from build123d import *

# Parameters (mm, degrees)
SKETCH1_W           = 54
SKETCH1_H           = 90
SKETCH1_W_2         = 38
SKETCH1_H_2         = 74
BOSS_EXTRUDE1_DEPTH = 40
CUT_EXTRUDE1_DEPTH  = 4.1
CUT_EXTRUDE2_DEPTH  = 0.5
CUT_EXTRUDE3_DEPTH  = 4.1
SKETCH7_R           = 4.1
CUT_EXTRUDE4_DEPTH  = 0.5
SKETCH8_W           = 54
SKETCH8_H           = 90
BOSS_EXTRUDE2_DEPTH = 2
SKETCH9_W           = 54
SKETCH9_H           = 90
BOSS_EXTRUDE3_DEPTH = 2


with BuildPart() as part:
    # Sketch1 → Boss-Extrude1 (new body)
    with BuildSketch(Plane.XY):
        with Locations((27, 45)):
            Rectangle(SKETCH1_W, SKETCH1_H)
        with Locations((27, 45)):
            Rectangle(SKETCH1_W_2, SKETCH1_H_2, mode=Mode.SUBTRACT)
    extrude(amount=BOSS_EXTRUDE1_DEPTH)

    # Sketch2 → Cut-Extrude1 (cut)
    with BuildSketch(Plane.ZY.offset(-46)):
        Polygon((25.888972746, 63), (22.944486373, 68.1), (17.055513627, 68.1), (14.111027254, 63), (17.055513627, 57.9), (22.944486373, 57.9), align=None)
        Polygon((25.888972746, 27), (22.944486373, 32.1), (17.055513627, 32.1), (14.111027254, 27), (17.055513627, 21.9), (22.944486373, 21.9), align=None)
    extrude(amount=-CUT_EXTRUDE1_DEPTH, mode=Mode.SUBTRACT)

    # Sketch5 → Cut-Extrude2 (cut)
    with BuildSketch(Plane.ZY.offset(-50.1)):
        Polygon((17.632863896, 22.9), (22.367136104, 22.9), (24.734272207, 27), (22.367136104, 31.1), (17.632863896, 31.1), (15.265727793, 27), align=None)
        Polygon((24.734272207, 63), (22.367136104, 67.1), (17.632863896, 67.1), (15.265727793, 63), (17.632863896, 58.9), (22.367136104, 58.9), align=None)
    extrude(amount=-CUT_EXTRUDE2_DEPTH, mode=Mode.SUBTRACT)

    # Sketch6 → Cut-Extrude3 (cut)
    with BuildSketch(Plane(origin=(8, 0, 0), x_dir=(0, 0, -1), z_dir=(1, 0, 0))):
        Polygon((-14.111027254, 63), (-17.055513627, 68.1), (-22.944486373, 68.1), (-25.888972746, 63), (-22.944486373, 57.9), (-17.055513627, 57.9), align=None)
        Polygon((-14.111027254, 27), (-17.055513627, 32.1), (-22.944486373, 32.1), (-25.888972746, 27), (-22.944486373, 21.9), (-17.055513627, 21.9), align=None)
    extrude(amount=-CUT_EXTRUDE3_DEPTH, mode=Mode.SUBTRACT)

    # Sketch7 → Cut-Extrude4 (cut)
    with BuildSketch(Plane(origin=(3.9, 0, 0), x_dir=(0, 0, -1), z_dir=(1, 0, 0))):
        with Locations((-20, 63)):
            Circle(SKETCH7_R)
        with Locations((-20, 27)):
            Circle(SKETCH7_R)
    extrude(amount=-CUT_EXTRUDE4_DEPTH, mode=Mode.SUBTRACT)

    # Sketch8 → Boss-Extrude2 (add)
    with BuildSketch(Plane.XY.offset(40)):
        with Locations((27, 45)):
            Rectangle(SKETCH8_W, SKETCH8_H)
    extrude(amount=BOSS_EXTRUDE2_DEPTH)

    # Sketch9 → Boss-Extrude3 (add)
    with BuildSketch(Plane(origin=(0, 0, 0), x_dir=(-1, 0, 0), z_dir=(0, 0, -1))):
        with Locations((-27, 45)):
            Rectangle(SKETCH9_W, SKETCH9_H)
    extrude(amount=BOSS_EXTRUDE3_DEPTH)


solid = part.part
Geometry: final body of the model. Coordinates: model frame, mm. Round coordinates to 2 decimals unless told otherwise and drop trailing zeros. Loops run counter-clockwise (first coordinate to the right, second up) from the corner with the lowest first, then second, coordinate; pieces in that order, holes last. Notation, with made-up numbers: M 18.25,20 L 48.25,20 A26 cw 48.25,55 Z; hole C 65.5,-4.5 d5. An arc over 180 degrees is marked long. Put each result on its own line as item: value. Start each with the question number.
(1) Section query D-D (y = 61.5). Return loops of the section in (x, z), then the cut area to 3 significant figures.
(2) Material intervals for line 1 along Y through (x, z) = (3.5, 20); line 2 along X through (y, z) = (34.5, 0.5); line 3 along Y through (x, z) = (20.5, 28), sorted ascending. Write a range as [from, to].
(3) Section query B-B (x = 22.5). Return loops of the section in (y, z), then the cut area to 3 significant figures.
(4) Draft query along Y for faces 1 (the face through (3.9, 23, 18)), 2 (the face through (0, 44, 20)). Return one class per face: +Y half, -Y half, draft (parallel to the pull), parting line (faces both ways), or undercut.
(5) Section query C-C (x = 48.5). Return loops of the section in (y, z).
(6) Section query A-A (z = 34). Return loops of the section in (x, y).
Findings below:
1. outline: M 0,-2 L 54,-2 L 54,42 L 0,42 Z; hole M 3.4,16.18 L 3.9,16.18 L 3.9,14.98 L 8,14.98 L 8,0 L 46,0 L 46,14.98 L 50.1,14.98 L 50.1,16.13 L 50.6,16.13 L 50.6,23.87 L 50.1,23.87 L 50.1,25.02 L 46,25.02 L 46,40 L 8,40 L 8,25.02 L 3.9,25.02 L 3.9,23.82 L 3.4,23.82 Z
1. area: 766 mm2
2. line 1: y = [0, 22.9], [31.1, 58.9], [67.1, 90]
2. line 2: x = [0, 8], [46, 54]
2. line 3: y = [0, 8], [82, 90]
3. outline: M 0,-2 L 90,-2 L 90,42 L 0,42 Z; hole M 8,0 L 82,0 L 82,40 L 8,40 Z
3. area: 1,000 mm2
4. face 1: undercut
4. face 2: draft
5. outline: M 0,-2 L 90,-2 L 90,42 L 0,42 Z; hole M 21.9,17.06 L 27,14.11 L 32.1,17.06 L 32.1,22.94 L 27,25.89 L 21.9,22.94 Z; hole M 57.9,17.06 L 63,14.11 L 68.1,17.06 L 68.1,22.94 L 63,25.89 L 57.9,22.94 Z
6. outline: M 0,0 L 54,0 L 54,90 L 0,90 Z; hole M 8,8 L 46,8 L 46,82 L 8,82 Z
